Input: part model. Units: mm. Frame: model coordinates. A direction names the side the tool comes from. Coordinates: 2 decimals unless noted, no trailing zeros. Order: outer loops, then holes, each group sorted by start corner. A loop starts at its lowest first (then second) coordinate and runs counter-clockwise, first axis right, second up. Notation, with made-up numbers: (13, 48) - (21, 48) arc R24 cw to (21, 83) - close; hole circle Ø3 at (-15, 16). An arc over 180 degrees is marked (long way). Use a Markdown table: item, result. Add a question column.
from build123d import *

# Parameters (mm, degrees)
SKETCH1_R           = 0.95
SKETCH1_R_2         = 0.7
BOSS_EXTRUDE1_DEPTH = 4
SKETCH2_W           = 16.2
SKETCH2_H           = 9.205
CUT_EXTRUDE1_DEPTH  = 2


with BuildPart() as part:
    # Sketch1 → Boss-Extrude1 (new body)
    with BuildSketch(Plane.XY):
        with BuildLine():
            Line((12.2, 4), (16.2, 4))
            Line((16.2, 4), (16.2, 2))
            ThreePointArc((16.2, 2), (15.614213562, 0.585786438), (14.2, 0))
            Line((14.2, 0), (2, 0))
            ThreePointArc((2, 0), (0.585786438, 0.585786438), (0, 2))
            Line((0, 2), (0, 4))
            Line((0, 4), (4, 4))
            Line((4, 4), (4, 6))
            Line((4, 6), (0, 6))
            Line((0, 6), (0, 9.205))
            ThreePointArc((0, 9.205), (1.464466094, 12.740533906), (5, 14.205))
            Line((5, 14.205), (11.2, 14.205))
            ThreePointArc((11.2, 14.205), (14.735533906, 12.740533906), (16.2, 9.205))
            Line((16.2, 9.205), (16.2, 6))
            Line((16.2, 6), (12.2, 6))
            Line((12.2, 6), (12.2, 4))
        make_face()
        with Locations((13.25, 2)):
            Circle(SKETCH1_R, mode=Mode.SUBTRACT)
        with Locations((13.2, 11.205)):
            Circle(SKETCH1_R_2, mode=Mode.SUBTRACT)
        with Locations((10.2, 7.75)):
            Circle(SKETCH1_R, mode=Mode.SUBTRACT)
        with Locations((6, 7.75)):
            Circle(SKETCH1_R, mode=Mode.SUBTRACT)
        with Locations((3, 11.205)):
            Circle(SKETCH1_R_2, mode=Mode.SUBTRACT)
        with Locations((2.95, 2)):
            Circle(SKETCH1_R, mode=Mode.SUBTRACT)
    extrude(amount=BOSS_EXTRUDE1_DEPTH)

    # Sketch2 → Cut-Extrude1 (cut)
    with BuildSketch(Plane(origin=(0, 0, 0), x_dir=(-1, 0, 0), z_dir=(0, 0, -1))):
        with Locations((-8.1, 4.6025)):
            Rectangle(SKETCH2_W, SKETCH2_H)
    extrude(amount=-CUT_EXTRUDE1_DEPTH, mode=Mode.SUBTRACT)


solid = part.part
1) Contact query for flat-ended pins moving along their axis: P1, Ø0.6, axis at x = 5, z = 0.5, coming from the -Y side (3 decimals); P2, Ø1, axis at x = 2.5, z = 2.5, coming from the +Y side; P3, Ø0.6, axis at x = 1.5, z = 3.5, coming from the +Y side. Output: stop coordinate, or through.
2) Reachability of faces 1 (the flat face through (2, 4, 3)), 2 (the cylindrical face through (10.076, 8.692, 2.986)), 3 (the flat face through (8, 5, 2)), 4 (the cylindrical face through (14.696, 12.779, 1.972)), 5 (the flat face through (14, 4, 3)) from +Z, -Z, +X, -X, +Y, -Y: full face, straight path, thin tool, end or side. Return the list, or none.
3) Pull-direction query (X, two-part tool) for faces 6 (the cylindrical face through (13.576, 11.795, 1.972)), 7 (the cylindrical face through (1.426, 12.701, 1.972)), 8 (the flat face through (8, 14.205, 2)); classes: pulls with the +X half, pulls with the -X half, needs draft (parallel to the pull), parting line crosses it, or undercut.
4) Material intervals for L1, parallel to X at y = 2, z = 2.45; L2, parallel to Y at x = 10.2, z = 2.4 (3 decimals); L3, parallel to X at y = 11.5, z = 1.5, sorted ascending.
5) Cut plane B-B (x = 10.2). Return the cut outline in (y, z) (3 decimals), and give its area (3 significant figures).
6) Cut plane C-C (x = 3). Return the cut outline in (y, z) (3 decimals), and give its area (3 significant figures).
7) Cut plane A-A (y = 7.75). Return the cut outline in (x, z).
8) Cut plane D-D (x = 5.75). Return the cut outline in (y, z) (3 decimals).
Computed:
| question | item | result |
|---|---|---|
| 1 | P1 | stops at y = 9.205 |
| 1 | P2 | stops at y = 13.79 |
| 1 | P3 | stops at y = 13.05 |
| 2 | face 1 | +Z, -Z, -X |
| 2 | face 2 | +Z, -Z |
| 2 | face 3 | -Z, +X, -X, -Y |
| 2 | face 4 | +Z, -Z, +X, +Y |
| 2 | face 5 | +Z, -Z, +X |
| 3 | face 6 | undercut |
| 3 | face 7 | pulls with the -X half |
| 3 | face 8 | needs draft |
| 4 | L1 | x = 0 to 2, 3.9 to 12.3, 14.2 to 16.2 |
| 4 | L2 | y = 0 to 6.8, 8.7 to 14.205 |
| 4 | L3 | x = 0.56 to 2.37, 3.63 to 12.57, 13.83 to 15.64 |
| 5 | outline | (0, 2) - (6.8, 2) - (6.8, 4) - (0, 4) - close; (8.7, 2) - (9.205, 2) - (9.205, 0) - (14.205, 0) - (14.205, 4) - (8.7, 4) - close |
| 5 | area | 34.6 mm2 |
| 6 | outline | (0, 2) - (1.051, 2) - (1.051, 4) - (0, 4) - close; (2.949, 2) - (4, 2) - (4, 4) - (2.949, 4) - close; (6, 2) - (9.205, 2) - (9.205, 0) - (10.505, 0) - (10.505, 4) - (6, 4) - close; (11.905, 0) - (13.788, 0) - (13.788, 4) - (11.905, 4) - close |
| 6 | area | 23.3 mm2 |
| 7 | outline | (0, 2) - (5.05, 2) - (5.05, 4) - (0, 4) - close; (6.95, 2) - (9.25, 2) - (9.25, 4) - (6.95, 4) - close; (11.15, 2) - (16.2, 2) - (16.2, 4) - (11.15, 4) - close |
| 8 | outline | (0, 2) - (6.833, 2) - (6.833, 4) - (0, 4) - close; (8.667, 2) - (9.205, 2) - (9.205, 0) - (14.205, 0) - (14.205, 4) - (8.667, 4) - close |
